Here's how the part is built. I have some questions about the finished solid (model axes, mm). Face numbers are marked on the shaded views. A direction names the side the tool comes from. Round coordinates to 2 decimals unless told otherwise and drop trailing zeros. Write each loop counter-clockwise with the first axis right and the second up, starting at its lowest first coordinate (ties: lowest second). Pieces come first, ordered by that corner, then holes. Notation, with made-up numbers: (-13, 34.25) -> (1, 34.25) arc R11 ccw to (1, 44.25) -> close; hole circle Ø8 at (30.5, 63.25). An arc over 180 degrees is marked (long way). Answer as CSV lines item,"result".
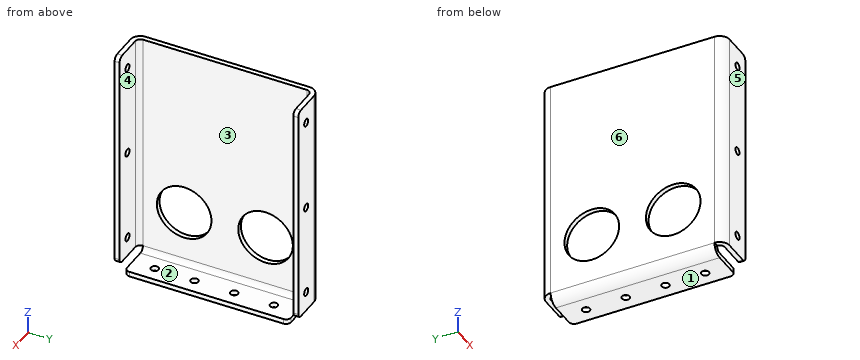
from build123d import *

# Parameters (mm, degrees)
BASE_FLANGE1_DEPTH = 142.875
EDGE_FLANGE1_DEPTH = 104.775
SKETCH9_R          = 17.4625
CUT_EXTRUDE1_DEPTH = 187.299736648
SKETCH10_R         = 2.4257
CUT_EXTRUDE2_DEPTH = 187.705118435
SKETCH11_R         = 2.4257
CUT_EXTRUDE3_DEPTH = 192.608027624
FILLET1_R          = 3.175


# Sheet-metal steps are written as plain solids
with BuildPart() as part:
    # Sketch1 → Base-Flange1 (new body)
    with BuildSketch(Plane.XY):
        with BuildLine():
            Line((25.4, 117.475), (6.35, 117.475))
            ThreePointArc((6.35, 117.475), (1.859871939, 115.615128061), (0, 111.125))
            Line((0, 111.125), (0, 6.35))
            ThreePointArc((0, 6.35), (1.859871939, 1.859871939), (6.35, 0))
            Line((6.35, 0), (25.4, 0))
            Line((25.4, 0), (25.4, 3.175))
            Line((25.4, 3.175), (6.35, 3.175))
            ThreePointArc((6.35, 3.175), (4.10493597, 4.10493597), (3.175, 6.35))
            Line((3.175, 6.35), (3.175, 111.125))
            ThreePointArc((3.175, 111.125), (4.10493597, 113.37006403), (6.35, 114.3))
            Line((6.35, 114.3), (25.4, 114.3))
            Line((25.4, 114.3), (25.4, 117.475))
        make_face()
    extrude(amount=BASE_FLANGE1_DEPTH)

    # Edge-Flange1 section (across the edge) → Edge-Flange1 (add)
    with BuildSketch(Plane(origin=(3.175, 6.35, -3.175), x_dir=(0, 0, 1), z_dir=(0, 1, 0))):
        with BuildLine():
            Line((-3.175, 3.175), (-3.175, 22.225))
            Line((-3.175, 22.225), (0, 22.225))
            Line((0, 22.225), (0, 3.175))
            ThreePointArc((0, 3.175), (0.92993597, 0.92993597), (3.175, 0))
            Line((3.175, 0), (3.175, -3.175))
            ThreePointArc((3.175, -3.175), (-1.315128061, -1.315128061), (-3.175, 3.175))
        make_face()
    extrude(amount=EDGE_FLANGE1_DEPTH)

    # Sketch9 → Cut-Extrude1 (cut, through all)
    with BuildSketch(Plane(origin=(3.175, 0, 0), x_dir=(0, 0, -1), z_dir=(1, 0, 0))):
        with Locations((-31.75, 84.7725)):
            Circle(SKETCH9_R)
        with Locations((-31.75, 32.7025)):
            Circle(SKETCH9_R)
    extrude(amount=-CUT_EXTRUDE1_DEPTH, mode=Mode.SUBTRACT)

    # Sketch10 → Cut-Extrude2 (cut, through all)
    with BuildSketch(Plane(origin=(0, 117.475, 0), x_dir=(1, 0, 0), z_dir=(0, 1, 0))):
        with Locations(Location((15.875, -71.4375, 0), (0, 0, 270))):
            Circle(SKETCH10_R)
        with Locations(Location((15.875, -130.175, 0), (0, 0, 270))):
            Circle(SKETCH10_R)
        with Locations(Location((15.875, -12.7, 0), (0, 0, 270))):
            Circle(SKETCH10_R)
    extrude(amount=-CUT_EXTRUDE2_DEPTH, mode=Mode.SUBTRACT)

    # Sketch11 → Cut-Extrude3 (cut, through all)
    with BuildSketch(Plane(origin=(0, 0, -6.35), x_dir=(-1, 0, 0), z_dir=(0, 0, -1))):
        with Locations((-15.875, 20.6375)):
            Circle(SKETCH11_R)
        with Locations((-15.875, 96.8375)):
            Circle(SKETCH11_R)
        with Locations((-15.875, 71.4375)):
            Circle(SKETCH11_R)
        with Locations((-15.875, 46.0375)):
            Circle(SKETCH11_R)
    extrude(amount=-CUT_EXTRUDE3_DEPTH, mode=Mode.SUBTRACT)

    # Fillet1
    fillet1_edges = [part.edges().sort_by_distance(p)[0] for p in [
        (25.4, 1.5875, 0),
        (25.4, 115.8875, 0),
        (25.4, 1.5875, 142.875),
        (25.4, 6.35, -4.7625),
        (25.4, 111.125, -4.7625),
        (25.4, 115.8875, 142.875),
    ]]
    fillet(fillet1_edges, radius=FILLET1_R)


solid = part.part
Item 1: I need wall thicknesses on L1, parallel to Y at x = 15.5, z = 65 (3 decimals); L2, parallel to Y at x = 2, z = 29.5; L3, parallel to Y at x = 1.25, z = 31.75 (3 decimals). Which ranges of each line are inside material? Lowest first, please.
Results found:
L1,"y = 0 to 3.175, 114.3 to 117.475"
L2,"y = 1.72 to 15.39, 50.02 to 67.46, 102.09 to 115.75"
L3,"y = 2.567 to 15.24, 50.165 to 67.31, 102.235 to 114.908"
Item 2: For the marked faces 1 and 2, which set-ups out of +Z, -Z, +X, -X, +Y, -Y let a thin tool reach every point of the face, with its end or its side?
Results found:
face 1,"-Z, +X, -X, +Y, -Y"
face 2,"+Z, +X, +Y, -Y"
Item 3: Suppose I cut it at D-D, the plane z = 12.7. List the corners of the cut face in (x, y) for me (3 decimals).
Results found:
outline,"(0, 6.35) arc R6.35 ccw to (6.35, 0) -> (13.449, 0) -> (13.449, 3.175) -> (6.35, 3.175) arc R3.175 cw to (3.175, 6.35) -> (3.175, 111.125) arc R3.175 cw to (6.35, 114.3) -> (13.449, 114.3) -> (13.449, 117.475) -> (6.35, 117.475) arc R6.35 ccw to (0, 111.125) -> close; (18.301, 0) -> (25.4, 0) -> (25.4, 3.175) -> (18.301, 3.175) -> close; (18.301, 114.3) -> (25.4, 114.3) -> (25.4, 117.475) -> (18.301, 117.475) -> close"
Item 4: Will these pins go through, and if not, where does the flat tip stop? pin 1 (15 mm diameter, centred on x = 14.5, y = 61.5, fed in from +Z) (3 decimals); pin 2 (3 mm diameter, centred on x = 15.88, y = 46.04, fed in from +Z); pin 3 (1.9 mm diameter, centred on x = 10, z = -4.5, fed in from +Y) (3 decimals); pin 4 (1.5 mm diameter, centred on y = 62.5, z = 117, fed in from +X) (3 decimals).
Results found:
pin 1,"stops at z = -3.175"
pin 2,"passes through"
pin 3,"stops at y = 111.125"
pin 4,"stops at x = 3.175"
Item 5: Suppose I cut it at A-A, the plane z = 31.75. List the corners of the cut face in (x, y) for me (3 decimals).
Results found:
outline,"(0, 6.35) arc R6.35 ccw to (6.35, 0) -> (25.4, 0) -> (25.4, 3.175) -> (6.35, 3.175) arc R3.175 cw to (3.175, 6.35) -> (3.175, 15.24) -> (0, 15.24) -> close; (0, 50.165) -> (3.175, 50.165) -> (3.175, 67.31) -> (0, 67.31) -> close; (0, 102.235) -> (3.175, 102.235) -> (3.175, 111.125) arc R3.175 cw to (6.35, 114.3) -> (25.4, 114.3) -> (25.4, 117.475) -> (6.35, 117.475) arc R6.35 ccw to (0, 111.125) -> close"
Item 6: Suppose I cut it at B-B, the plane y = 78.5. List the corners of the cut face in (x, z) for me (3 decimals).
Results found:
outline,"(0, 0) arc R6.35 ccw to (6.35, -6.35) -> (25.4, -6.35) -> (25.4, -3.175) -> (6.35, -3.175) arc R3.175 cw to (3.175, 0) -> (3.175, 15.453) -> (0, 15.453) -> close; (0, 48.047) -> (3.175, 48.047) -> (3.175, 142.875) -> (0, 142.875) -> close"
Item 7: Suppose I cut it at C-C, the plane x = 9. List the corners of the cut face in (y, z) for me (3 decimals).
Results found:
outline,"(0, 0) -> (3.175, 0) -> (3.175, 142.875) -> (0, 142.875) -> close; (6.35, -6.35) -> (111.125, -6.35) -> (111.125, -3.175) -> (6.35, -3.175) -> close; (114.3, 0) -> (117.475, 0) -> (117.475, 142.875) -> (114.3, 142.875) -> close"
Item 8: If we mould it in two halves opening along Y, with no side actions, what happens to the marked faces 3, 4, 5 and 6? For each: pulls with the +Y half, pulls with the -Y half, needs draft (parallel to the pull), parting line crosses it, or undercut.
Results found:
face 3,"undercut"
face 4,"undercut"
face 5,"pulls with the -Y half"
face 6,"needs draft"
